from build123d import *

# Parameters (mm, degrees)
F1_DEPTH  = 7.9375
F3_DEPTH  = 15.875
F4_W      = 71.9558009878
F4_H      = 13.6753677544
F5_DEPTH  = 87.884
F7_DEPTH  = 84.582
F8_R      = 5.5626
F9_DEPTH  = 25.4
F10_R     = 28.575
F11_DEPTH = 63.7286
F12_R     = 19.05
F13_DEPTH = 95.758
F15_DEPTH = 63.5


with BuildPart() as f1:
    # F0 (on Front) → F1 (new body, symmetric)
    with BuildSketch(Plane.XZ):
        Polygon((0, 63.5), (0, 0), (50.8, 0), (50.8, 63.7060776353), align=None)
    extrude(amount=F1_DEPTH, both=True)

    # F2 (on face) → F3 (join, symmetric)
    with BuildSketch(Plane.XZ.offset(7.9375)):
        with BuildLine():
            ThreePointArc((-39.632043346, 20.4206049765), (-26.9943232846, 20.5270910991), (-20.706004086, 31.4897709403))
            ThreePointArc((-20.706004086, 31.4897709403), (-27.0842562365, 42.5045566453), (-39.8123826888, 42.4555501282))
            ThreePointArc((-39.8123826888, 42.4555501282), (-46.1055787727, 31.3858345367), (-39.632043346, 20.4206049765))
        make_face()
        with BuildLine():
            ThreePointArc((-39.8123826888, 42.4555501282), (-27.0842562365, 42.5045566453), (-20.706004086, 31.4897709403))
            ThreePointArc((-20.706004086, 31.4897709403), (-26.9943232846, 20.5270910991), (-39.632043346, 20.4206049765))
            Line((-39.632043346, 20.4206049765), (-6.22603926, 1.6308340362))
            ThreePointArc((-6.22603926, 1.6308340362), (-6.4116808014, 23.6626798412), (12.7, 12.7))
            Line((12.7, 12.7), (12.7, 51.0060776353))
            ThreePointArc((12.7, 51.0060776353), (-6.3217478495, 39.9912919303), (-6.4063786028, 61.9718568232))
            Line((-6.4063786028, 61.9718568232), (-39.8123826888, 42.4555501282))
        make_face()
        with BuildLine():
            ThreePointArc((12.7, 51.0060776353), (6.3217478495, 62.0208633403), (-6.4063786028, 61.9718568232))
            ThreePointArc((-6.4063786028, 61.9718568232), (-6.3217478495, 39.9912919303), (12.7, 51.0060776353))
        make_face()
        with BuildLine():
            ThreePointArc((12.7, 12.7), (-6.4116808014, 23.6626798412), (-6.22603926, 1.6308340362))
            ThreePointArc((-6.22603926, 1.6308340362), (6.4116808014, 1.7373201588), (12.7, 12.7))
        make_face()
    extrude(amount=F3_DEPTH, both=True)

    # F4 (on face) → F5 (cut)
    with BuildSketch(Plane(origin=(-0.7994989556, 0, -1.4214151659), x_dir=(0.8715878712, 0, -0.4902393118), z_dir=(-0.4902393118, 0, -0.8715878712))):
        with Locations((-20.4755323939, 19.3995043051)):
            Rectangle(F4_W, F4_H)
    extrude(amount=-F5_DEPTH, mode=Mode.SUBTRACT)

    # F6 (on Top) → F7 (cut)
    with BuildSketch(Plane.XY):
        Polygon((-39.6329276264, -12.583178468), (-41.4357371628, -12.583178468), (-46.0986830294, -12.583178468), (-46.0986830294, -26.8648453057), (-39.6329276264, -26.8648453057), align=None)
    extrude(amount=F7_DEPTH, mode=Mode.SUBTRACT)

    # F8 (on face) → F9 (cut)
    with BuildSketch(Plane.XZ.offset(12.5618204279)):
        with Locations((0, 51.0060776353)):
            Circle(F8_R)
        with Locations((0, 12.7)):
            Circle(F8_R)
        with Locations((-33.406004086, 31.4897709403)):
            Circle(F8_R)
    extrude(amount=-F9_DEPTH, mode=Mode.SUBTRACT)

    # F10 (on face) → F11 (join)
    with BuildSketch(Plane(origin=(-0.2575928051, 0, 63.4989550371), x_dir=(0.9999917719, 0, 0.004056613), z_dir=(-0.004056613, 0, 0.9999917719))):
        with Locations((51.0580129149, 20.6375)):
            Circle(F10_R)
    extrude(amount=-F11_DEPTH)

    # F12 (on face) → F13 (cut)
    with BuildSketch(Plane(origin=(-0.2575928051, 0, 63.4989550371), x_dir=(0.9999917719, 0, 0.004056613), z_dir=(-0.004056613, 0, 0.9999917719))):
        with Locations((51.0580129149, 20.6375)):
            Circle(F12_R)
    extrude(amount=-F13_DEPTH, mode=Mode.SUBTRACT)

    # F14 (on face) → F15 (join)
    with BuildSketch(Plane(origin=(-0.2575928051, 0, 63.4989550371), x_dir=(0.9999917719, 0, 0.004056613), z_dir=(-0.004056613, 0, 0.9999917719))):
        with BuildLine():
            Line((13.9709103513, 7.9375), (12.2397709638, 7.9375))
            ThreePointArc((12.2397709638, 7.9375), (13.1053406575, 7.8980898133), (13.9709103513, 7.9375))
        make_face()
        with BuildLine():
            ThreePointArc((22.5536784489, 18.6291320929), (20.5331210195, 11.4603971418), (13.9709103513, 7.9375))
            Line((13.9709103513, 7.9375), (25.4603445641, 7.9375))
            Line((25.4603445641, 7.9375), (22.5536784489, 18.6291320929))
        make_face()
    extrude(amount=-F15_DEPTH)


solid = f1.part
Can you work these out from the model? Positions are in its coordinate system, mm. A direction names the side the tool comes from. Give positions to 0.01 mm unless a question says otherwise; leave off trailing zeros. Loops run counter-clockwise (first coordinate to the right, second up) from the corner with the lowest first, then second, coordinate; pieces in that order, holes last. Notation, with made-up numbers: M 44,12.25 L 69,12.25 A17 ccw 69,34.25 Z; hole C 48.25,-31 d2. An arc over 180 degrees is marked long. One line per item, written item: value. Start each with the question number.
1) Thinking about a two-plate mould opening in Z: for faces 1 (the face through (-30.416, -2.456, 36.18)), 2 (the face through (-0.72, -2.46, 56.52)), 3 (the face through (-44, -12.583, 38)), 4 (the face through (-23.163, -2.456, 11.157)), which applies, +Z half, -Z half, draft (parallel to the pull), parting line (faces both ways), or undercut?
2) If I drill on line 1 (Z direction, x = 0, y = -4); line 2 (Y direction, x = 50, z = 16.5); line 3 (X direction, y = 5, z = 51.5), over which ranges is the centre line in solid material (lowest first)? Write a range as [from, to].
3) If we section it at A-A, the plane y = -1.5: Write out the boundary of the cut face in (x, z), and give its area (3 significant figures).
4) If we section it at B-B, the plane z = 29.5: Give the number of separate pieces and of enclosed holes in the cut face, and give its area (3 significant figures).
5) I'm going to push flat-ended pins straight in: pin 1 (4 mm diameter, centred on x = -1, z = 30.5, fed in from -Y); pin 2 (13 mm diameter, centred on x = 0, z = 51.01, fed in from +Y); pin 3 (6 mm diameter, centred on x = 23.5, y = -1.5, fed in from +Z); pin 4 (10 mm diameter, centred on x = 0, z = 12.7, fed in from +Y). Where does each tip first touch, or does it pass through?
6) On a 3-axis mill with a long thin cutter (end or side, diameter ignored), from which of +Z, -Z, +X, -X, +Y, -Y can I reach the whole of each face in a straight line? I mean faces 5 (the face through (19, 0, 0)), 6 (the face through (0.878, -4.733, 63.676)), 7 (the face through (12.7, -10, 32)), 8 (the face through (46.8, 2.04, 32.27)). Say none if no direction works.
Completed:
1. face 1: undercut
1. face 2: undercut
1. face 3: draft
1. face 4: -Z half
2. line 1: z = [0, 7.14], [18.26, 45.44], [56.57, 63.71]
2. line 2: y = [-7.94, 1.61], [39.66, 49.2]
2. line 3: x = [-24.33, -5.54], [5.54, 39.97], [61.73, 74.77]
3. outline: M -39.81,42.46 A12.7 ccw -39.63,20.42 L -6.23,1.63 A12.7 ccw 0,0 L 32.99,0 L 32.99,-0.1 L 69.13,0.05 L 68.87,63.78 L 2.23,63.51 A12.7 ccw -6.41,61.97 Z; hole C -33.41,31.49 d11.13; hole C 0,12.7 d11.13; hole C 0,51.01 d11.13
3. area: 5,970 mm^2
4. separate pieces: 2
4. enclosed holes: 1
4. area: 2,760 mm^2
5. pin 1: stops at y = -12.56
5. pin 2: stops at y = 7.94
5. pin 3: stops at z = 63.61
5. pin 4: passes through
6. face 5: -Z, -X, -Y
6. face 6: +Z, -Y
6. face 7: +Z, -Z, +X, -Y
6. face 8: none
